```python
from build123d import *

# Parameters (mm, degrees)
SKETCH_1_W          = 30
SKETCH_1_H          = 10
SKETCH_1_W_2        = 26
SKETCH_1_H_2        = 6
EXTRUDE_1_DEPTH     = 67
SKETCH_2_R          = 1.5
CUT_EXTRUDE_1_DEPTH = 70.382995035


with BuildPart() as part:
    # 草图1 → 凸台-拉伸1 (new, symmetric)
    with BuildSketch(Plane(origin=(0, 0, 0), x_dir=(1, 0, 0), z_dir=(0, 1, 0))):
        Rectangle(SKETCH_1_W, SKETCH_1_H)
        Rectangle(SKETCH_1_W_2, SKETCH_1_H_2, mode=Mode.SUBTRACT)
    extrude(amount=EXTRUDE_1_DEPTH, both=True)

    # 草图2 → 切除-拉伸1 (cut, through all)
    with BuildSketch(Plane.XY.offset(5)):
        with Locations((-10, 62)):
            Circle(SKETCH_2_R)
        with Locations((0, 62)):
            Circle(SKETCH_2_R)
        with Locations((10, 62)):
            Circle(SKETCH_2_R)
        with Locations((-5, 25)):
            Circle(SKETCH_2_R)
        with Locations((-5, 15)):
            Circle(SKETCH_2_R)
        with Locations((5, 15)):
            Circle(SKETCH_2_R)
        with Locations((5, 25)):
            Circle(SKETCH_2_R)
        with Locations(Location((-5, -15, 0), (0, 0, 180))):
            Circle(SKETCH_2_R)
        with Locations(Location((5, -15, 0), (0, 0, 180))):
            Circle(SKETCH_2_R)
        with Locations(Location((5, -25, 0), (0, 0, 180))):
            Circle(SKETCH_2_R)
        with Locations(Location((-5, -25, 0), (0, 0, 180))):
            Circle(SKETCH_2_R)
        with Locations(Location((-10, -62, 0), (0, 0, 180))):
            Circle(SKETCH_2_R)
        with Locations(Location((0, -62, 0), (0, 0, 180))):
            Circle(SKETCH_2_R)
        with Locations(Location((10, -62, 0), (0, 0, 180))):
            Circle(SKETCH_2_R)
    extrude(amount=-CUT_EXTRUDE_1_DEPTH, mode=Mode.SUBTRACT)


solid = part.part
```
The listing builds one solid part. Answer for the finished solid, in the listing's coordinates (mm). A direction names the side the tool comes from. Round coordinates to 2 decimals unless told otherwise and drop trailing zeros. Loops run counter-clockwise (first coordinate to the right, second up) from the corner with the lowest first, then second, coordinate; pieces in that order, holes last. Notation, with made-up numbers: (53, 20.5) - (59, 20.5) arc R21 cw to (59, 57.5) - close; hole circle Ø10 at (-27.5, 19.5). An arc over 180 degrees is marked (long way). Use one line per item in the form item = value. Start each with the question number.
1. Given pin 1 Ø2.5 at (x, y) = (5, 25) entering from +Z, flat-ended and moving along its own axis, determine where the tip first touches the part or whether it passes through.
2. Consider line 1 (X direction, y = -62, z = -4.25); line 2 (Y direction, x = 5, z = -3.9); line 3 (X direction, y = -15, z = 3.65). Determine where each line is inside the solid, lowest interval first. Write a range as [from, to].
3. For a pull along Z with two mould halves and no side action, classify faces 1 (the face through (-13, 1, 0)), 2 (the face through (6.386, 14.425, 4.014)) as pulls with the +Z half, pulls with the -Z half, needs draft (parallel to the pull), parting line crosses it, or undercut.
4. The part is cut by section B-B on x = 0. Determine the outline of the cut face in (y, z), then the cut area to 3 significant figures.
5. The part is cut by section D-D on z = -1. Determine the outline of the cut face in (x, y), then the cut area to 3 significant figures.
6. The part is cut by section C-C on y = -15. Determine the outline of the cut face in (x, z).
7. The part is cut by section A-A on y = 11.5. Determine the outline of the cut face in (x, z), then the cut area to 3 significant figures.
8. A tool of negligible diameter and unlimited length cuts with its end or side. For faces 3 (the face through (0, 1, -3)), 4 (the face through (-0.2, -67, -3.4)), from which of +Z, -Z, +X, -X, +Y, -Y can it reach the whole face along a straight path? Write none if from no direction.
Geometry check:
q1.pin_1 = through
q2.line_1 = [-15, -11.5], [-8.5, -1.5], [1.5, 8.5], [11.5, 15]
q2.line_2 = [-67, -26.5], [-23.5, -16.5], [-13.5, 13.5], [16.5, 23.5], [26.5, 67]
q2.line_3 = [-15, -6.5], [-3.5, 3.5], [6.5, 15]
q3.face_1 = undercut
q3.face_2 = needs draft
q4.outline = (-67, -5) - (-63.5, -5) - (-63.5, -3) - (-67, -3) - close; (-67, 3) - (-63.5, 3) - (-63.5, 5) - (-67, 5) - close; (-60.5, -5) - (60.5, -5) - (60.5, -3) - (-60.5, -3) - close; (-60.5, 3) - (60.5, 3) - (60.5, 5) - (-60.5, 5) - close; (63.5, -5) - (67, -5) - (67, -3) - (63.5, -3) - close; (63.5, 3) - (67, 3) - (67, 5) - (63.5, 5) - close
q4.area = 512 mm^2
q5.outline = (-15, -67) - (-13, -67) - (-13, 67) - (-15, 67) - close; (13, -67) - (15, -67) - (15, 67) - (13, 67) - close
q5.area = 536 mm^2
q6.outline = (-15, -5) - (-6.5, -5) - (-6.5, -3) - (-13, -3) - (-13, 3) - (-6.5, 3) - (-6.5, 5) - (-15, 5) - close; (-3.5, -5) - (3.5, -5) - (3.5, -3) - (-3.5, -3) - close; (-3.5, 3) - (3.5, 3) - (3.5, 5) - (-3.5, 5) - close; (6.5, -5) - (15, -5) - (15, 5) - (6.5, 5) - (6.5, 3) - (13, 3) - (13, -3) - (6.5, -3) - close
q7.outline = (-15, -5) - (15, -5) - (15, 5) - (-15, 5) - close; hole (-13, -3) - (13, -3) - (13, 3) - (-13, 3) - close
q7.area = 144 mm^2
q8.face_3 = +Y, -Y
q8.face_4 = +Z, -Z, +X, -X, -Y
